Check sheet for the modelled part. Datum: model origin and axes. Units: mm. A direction names the side the tool comes from. Round coordinates to 2 decimals unless told otherwise and drop trailing zeros. Write each loop counter-clockwise with the first axis right and the second up, starting at its lowest first coordinate (ties: lowest second). Pieces come first, ordered by that corner, then holes. Notation, with made-up numbers: M -17,1 L -7,1 A16 ccw -7,25 Z; hole C 73,13 d2. An arc over 180 degrees is marked long. Answer in a Markdown table with one row per item.
Autodesk Inventor part; units mm, degrees
ref_plane "YZ Plane" through (0, 0, 0) normal (1, 0, 0) x (0, 1, 0)
ref_plane "XZ Plane" through (0, 0, 0) normal (0, 1, 0) x (-1, 0, 0)
ref_plane "XY Plane" through (0, 0, 0) normal (0, 0, 1) x (1, 0, 0)
sketch "Sketch1" plane through (0, 0, 0) normal (0, 0, 1) x (1, 0, 0)
  line L0 (0, 0) -> (25.4, 0)
  line L1 (25.4, 0) -> (25.4, 25.4)
  line L2 (25.4, 25.4) -> (0, 25.4)
  line L3 (0, 25.4) -> (0, 0)
  line L4 (1.5875, 23.8125) -> (23.6267, 23.8125)
  line L5 (23.6267, 23.8125) -> (23.6267, 2.0041)
  line L6 (23.6267, 2.0041) -> (1.5875, 2.0041)
  line L7 (1.5875, 2.0041) -> (1.5875, 23.8125)
  dimension "d0" = 25.4
  dimension "d1" = 25.4
  dimension "d2" = 1.5875
  dimension "d3" = 1.5875
extrude "Extrusion1" add sketch "Sketch1" along normal blind 203.2
sketch "Sketch2" plane through (0, 25.4, 0) normal (0, 1, 0) x (1, 0, 0)
  line L0 (25.4, 0) -> (0, 0)
  line L1 (25.4, 0) -> (25.4, -203.2)
  point P0 (12.7, -12.7)
  point P1 (12.7, -38.1)
  point P2 (12.7, -63.5)
  point P3 (12.7, -88.9)
  point P4 (12.7, -114.3)
  point P5 (12.7, -139.7)
  point P6 (12.7, -165.1)
  point P7 (12.7, -190.5)
  point P8 (12.7, -215.9)
  point P9 (12.7, -241.3)
  point P10 (12.7, -266.7)
  point P11 (12.7, -292.1)
  point P12 (12.7, -317.5)
  point P13 (12.7, -342.9)
  point P14 (12.7, -368.3)
  dimension "d6" = 12.7
  dimension "d7" = 12.7
  dimension "d10" = 25.4
hole "Hole1" at (12.7, 25.4, 12.7) at (12.7, 25.4, 38.1) at (12.7, 25.4, 63.5) at (12.7, 25.4, 88.9) at (12.7, 25.4, 114.3) at (12.7, 25.4, 139.7) at (12.7, 25.4, 165.1) at (12.7, 25.4, 190.5) at (12.7, 25.4, 215.9) at (12.7, 25.4, 241.3) at (12.7, 25.4, 266.7) at (12.7, 25.4, 292.1) at (12.7, 25.4, 317.5) at (12.7, 25.4, 342.9) at (12.7, 25.4, 368.3) direction (0, -1, 0) diameter 2.54 depth 25.4 tip angle 118
properties part number "Drive Rail 1 upright 2"
1. Scan lines: L1, parallel to X at y = 16, z = 59; L2, parallel to Y at x = 8.25, z = 63; L3, parallel to X at y = 1.15, z = 139.7. Record each from-to range of solid material in increasing order.
Found:
| item | result |
|---|---|
| L1 | x = 0 to 1.59, 23.63 to 25.4 |
| L2 | y = 0 to 2, 23.81 to 25.4 |
| L3 | x = 0 to 11.43, 13.97 to 25.4 |
2. Access from +Z, -Z, +X, -X, +Y, -Y to the whole of each face (thin tool, end or side, straight path). Record for faces 4 (the face through (12, 23.812, 100)), 5 (the face through (24, 13, 0)).
Found:
| item | result |
|---|---|
| face 4 | +Z, -Z |
| face 5 | -Z, +X, -X, +Y, -Y |
3. Section check A-A, the plane x = 18. Record the cut outline in (y, z).
Found:
| item | result |
|---|---|
| outline | M 0,0 L 2,0 L 2,203.2 L 0,203.2 Z; M 23.81,0 L 25.4,0 L 25.4,203.2 L 23.81,203.2 Z |
4. Section check C-C, the plane y = 8. Record the cut outline in (x, z).
Found:
| item | result |
|---|---|
| outline | M 0,0 L 1.59,0 L 1.59,203.2 L 0,203.2 Z; M 23.63,0 L 25.4,0 L 25.4,203.2 L 23.63,203.2 Z |
5. Draft check along Y on faces 1 (the face through (13, 25.4, 100)), 2 (the face through (0, 13, 100)), 3 (the face through (23.627, 13, 100)). Enter one of: +Y half, -Y half, draft (parallel to the pull), parting line (faces both ways), or undercut.
Found:
| item | result |
|---|---|
| face 1 | +Y half |
| face 2 | draft |
| face 3 | undercut |
6. Section check B-B, the plane z = 111. Record the cut outline in (x, y), and give its area (3 significant figures).
Found:
| item | result |
|---|---|
| outline | M 0,0 L 25.4,0 L 25.4,25.4 L 0,25.4 Z; hole M 1.59,2 L 23.63,2 L 23.63,23.81 L 1.59,23.81 Z |
| area | 165 mm2 |
